Could you check a few things on this model? Use its own coordinates, in mm. A direction names the side the tool comes from. Give positions to 0.01 mm unless a question says otherwise; leave off trailing zeros. Write each loop counter-clockwise with the first axis right and the second up, starting at its lowest first coordinate (ties: lowest second). Pieces come first, ordered by that corner, then holes. Notation, with made-up numbers: (-14.5, 44) - (-8.5, 44) arc R14 ccw to (-8.5, 52) - close; hole circle Ø8 at (-18, 20.25). An arc over 180 degrees is marked (long way). Write item = value, one per line.
from build123d import *

# Parameters (mm, degrees)
SKETCH2_W           = 70
SKETCH2_H           = 100
BOSS_EXTRUDE3_DEPTH = 12.7


with BuildPart() as part:
    # Sketch2 → Boss-Extrude3 (new body)
    with BuildSketch(Plane.XY):
        with BuildLine():
            Line((-200, -230.044545372), (-135.055496126, -300))
            Line((-135.055496126, -300), (-125.080405008, -300))
            Line((-125.080405008, -300), (-125.080405008, -220))
            Line((-125.080405008, -220), (124.919594992, -220))
            Line((124.919594992, -220), (124.919594992, -300))
            Line((124.919594992, -300), (134.911595754, -300))
            Line((134.911595754, -300), (200, -230.044545372))
            Line((200, -230.044545372), (200, 120.049170717))
            Line((200, 120.049170717), (28.699194546, 274.177780708))
            ThreePointArc((28.699194546, 274.177780708), (0, 312.915986038), (-28.699194546, 274.177780708))
            Line((-28.699194546, 274.177780708), (-200, 120.049170717))
            Line((-200, 120.049170717), (-200, -230.044545372))
        make_face()
        Polygon((-187.3, -198.731620565), (-187.3, -120), (-101.303698117, -120), align=None, mode=Mode.SUBTRACT)
        Polygon((-177.851600054, -207.3), (-91.979918019, -128.682471814), (-9.219885484, -207.3), align=None, mode=Mode.SUBTRACT)
        Polygon((-0.473030641, -198.092257044), (-82.680114516, -120), (82.015084133, -120), align=None, mode=Mode.SUBTRACT)
        with Locations((-152.3, -57.3)):
            Rectangle(SKETCH2_W, SKETCH2_H, mode=Mode.SUBTRACT)
        Polygon((-71.265160823, 50.024585359), (-45.501144454, 5.4), (-187.3, 5.4), (-187.3, 50.024585359), align=None, mode=Mode.SUBTRACT)
        Polygon((-104.6, -7.3), (-9.189123593, -7.3), (-104.6, -98.514987005), align=None, mode=Mode.SUBTRACT)
        Polygon((177.8939034, -207.3), (9.189123593, -207.3), (90.58572411, -127.795746586), (161.581783291, -192.372871222), align=None, mode=Mode.SUBTRACT)
        Polygon((187.3, -198.092257044), (98.567023769, -120), (187.3, -120), align=None, mode=Mode.SUBTRACT)
        Polygon((-95.410876407, -107.3), (-0.412987416, -16.479838441), (30.242078983, -44.997134394), (95.410876407, -107.3), align=None, mode=Mode.SUBTRACT)
        Polygon((9.189123593, -7.3), (104.6, -7.3), (104.6, -98.514987005), align=None, mode=Mode.SUBTRACT)
        with Locations((152.3, -57.3)):
            Rectangle(SKETCH2_W, SKETCH2_H, mode=Mode.SUBTRACT)
        Polygon((-45.501144454, 107.349170717), (-71.265160823, 62.724585359), (-187.3, 62.724585359), (-187.3, 107.349170717), align=None, mode=Mode.SUBTRACT)
        Polygon((-112.679699791, 181.531958935), (-27.970761031, 120.049170717), (-181.012575458, 120.049170717), align=None, mode=Mode.SUBTRACT)
        Polygon((-103.026071592, 190.217850935), (-6.35, 190.217850935), (-6.35, 120.049170717), align=None, mode=Mode.SUBTRACT)
        with BuildLine():
            Line((-6.35, 253.595728536), (-6.35, 202.917850935))
            Line((-6.35, 202.917850935), (-88.911104686, 202.917850935))
            Line((-88.911104686, 202.917850935), (-22.301550494, 262.85007351))
            ThreePointArc((-22.301550494, 262.85007351), (-15.054519642, 256.966777219), (-6.35, 253.595728536))
        make_face(mode=Mode.SUBTRACT)
        Polygon((29.439464567, 5.383936982), (-29.439464567, 5.383936982), (-58.878929133, 56.374585359), (-29.439464567, 107.365233736), (29.439464567, 107.365233736), (58.878929133, 56.374585359), align=None, mode=Mode.SUBTRACT)
        Polygon((187.3, 5.4), (45.501144454, 5.4), (71.265160823, 50.024585359), (187.3, 50.024585359), align=None, mode=Mode.SUBTRACT)
        Polygon((187.3, 107.349170717), (187.3, 62.724585359), (71.265160823, 62.724585359), (45.501144454, 107.349170717), align=None, mode=Mode.SUBTRACT)
        Polygon((6.35, 120.049170717), (6.35, 190.217850935), (103.026071592, 190.217850935), align=None, mode=Mode.SUBTRACT)
        with BuildLine():
            Line((6.35, 202.917850935), (6.35, 253.595728536))
            ThreePointArc((6.35, 253.595728536), (15.054519642, 256.966777219), (22.301550494, 262.85007351))
            Line((22.301550494, 262.85007351), (88.911104686, 202.917850935))
            Line((88.911104686, 202.917850935), (6.35, 202.917850935))
        make_face(mode=Mode.SUBTRACT)
        Polygon((181.012575458, 120.049170717), (27.970761031, 120.049170717), (112.679699791, 181.531958935), align=None, mode=Mode.SUBTRACT)
    extrude(amount=BOSS_EXTRUDE3_DEPTH)


solid = part.part
1. If we section it at A-A, the plane y = 134: Please give me the cut outline in (x, z).
Filled sheet:
outline = (-184.49, 0) - (-165.51, 0) - (-165.51, 12.7) - (-184.49, 12.7) - close; (-47.19, 0) - (-25.57, 0) - (-25.57, 12.7) - (-47.19, 12.7) - close; (-6.35, 0) - (6.35, 0) - (6.35, 12.7) - (-6.35, 12.7) - close; (25.57, 0) - (47.19, 0) - (47.19, 12.7) - (25.57, 12.7) - close; (165.51, 0) - (184.49, 0) - (184.49, 12.7) - (165.51, 12.7) - close
2. I need wall thicknesses on line 1 (X direction, y = 26, z = 7); line 2 (X direction, y = -131, z = 5.25); line 3 (X direction, y = -20.5, z = 5). Which ranges of each line are inside material? Lowest first, please.
Filled sheet:
line_1 = -200 to -187.3, -57.39 to -41.34, 41.34 to 57.39, 187.3 to 200
line_2 = -200 to -187.3, -113.32 to -94.51, -89.54 to -71.1, 70.4 to 87.31, 94.11 to 111.07, 187.3 to 200
line_3 = -200 to -187.3, -117.3 to -104.6, -23 to -4.62, 3.91 to 23, 104.6 to 117.3, 187.3 to 200
3. If we section it at D-D, the plane y = -82.5: Please give me the cut outline in (x, z).
Filled sheet:
outline = (-200, 0) - (-187.3, 0) - (-187.3, 12.7) - (-200, 12.7) - close; (-117.3, 0) - (-104.6, 0) - (-104.6, 12.7) - (-117.3, 12.7) - close; (-87.85, 0) - (-69.47, 0) - (-69.47, 12.7) - (-87.85, 12.7) - close; (69.47, 0) - (87.85, 0) - (87.85, 12.7) - (69.47, 12.7) - close; (104.6, 0) - (117.3, 0) - (117.3, 12.7) - (104.6, 12.7) - close; (187.3, 0) - (200, 0) - (200, 12.7) - (187.3, 12.7) - close
4. If we section it at C-C, the plane z = 2.5: Count the separate pieces of the cut face and the enclosed holes in it, and give its area (3 significant figures).
Filled sheet:
separate_pieces = 1
enclosed_holes = 21
area = 68,700 mm2
5. For pin 1 (4 mm diameter, centred on x = -55.5, z = 5, fed in from +Y); pin 2 (3 mm diameter, centred on y = 204, z = 6, fed in from +X); pin 3 (4 mm diameter, centred on x = 77.5, z = 7.5, fed in from -Y), each with a flat end and sliding along its axis, tell me the tip position at first contact or that it passes through.
Filled sheet:
pin_1 = 251.86
pin_2 = 108.36
pin_3 = -220
6. Which directions (+Z, -Z, +X, -X, +Y, -Y) give clear straight access to the entire face, cutting with the end or side of a thin tool? Please do faces 1 (the face through (-125.08, -261, 6)), 2 (the face through (167, -265.51, 6.26)), 3 (the face through (152, -107.3, 6)).
Filled sheet:
face_1 = +Z, -Z, -Y
face_2 = +Z, -Z, +X, -Y
face_3 = +Z, -Z
7. Thinking about a two-plate mould opening in Y: for faces 4 (the face through (29, -38, 0)), 5 (the face through (-167.982, -264.533, 6.261)), 6 (the face through (55.14, 233.303, 6.261)), which applies, pulls with the +Y half, pulls with the -Y half, needs draft (parallel to the pull), parting line crosses it, or undercut?
Filled sheet:
face_4 = needs draft
face_5 = pulls with the -Y half
face_6 = undercut
8. If we section it at B-B, the plane y = 70.5: Please give me the cut outline in (x, z), and give its area (3 significant figures).
Filled sheet:
outline = (-200, 0) - (-187.3, 0) - (-187.3, 12.7) - (-200, 12.7) - close; (-66.78, 0) - (-50.72, 0) - (-50.72, 12.7) - (-66.78, 12.7) - close; (50.72, 0) - (66.78, 0) - (66.78, 12.7) - (50.72, 12.7) - close; (187.3, 0) - (200, 0) - (200, 12.7) - (187.3, 12.7) - close
area = 730 mm2
